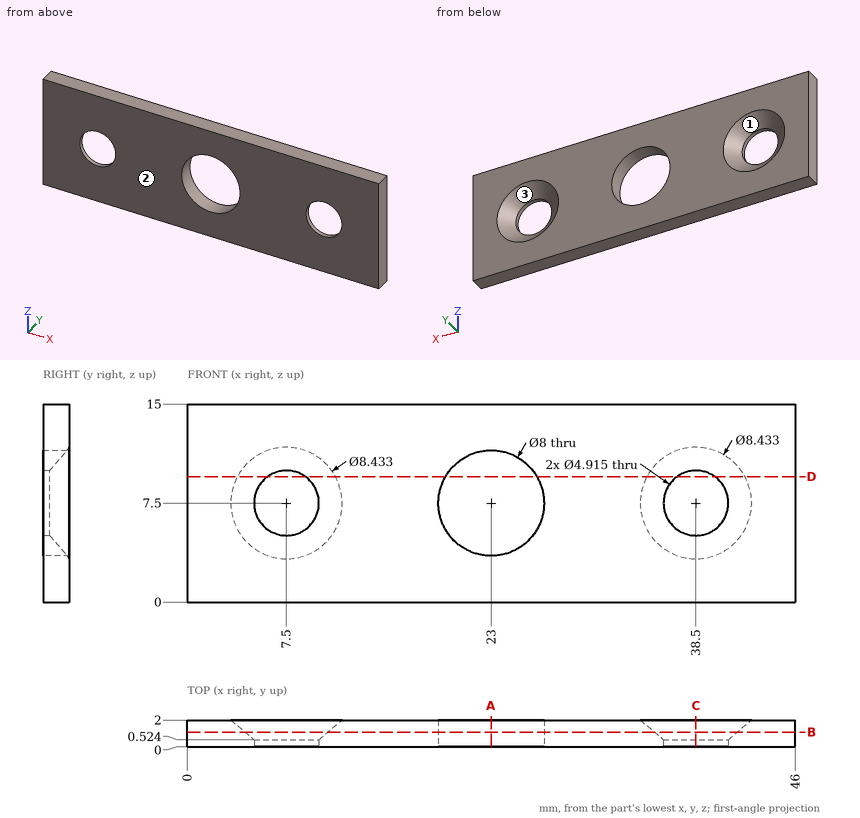
Geometry check sheet. Reference: drawing and pictorial views, mm from the part's lowest x, y, z. Give positions to 0.01 mm unless a question says otherwise; leave off trailing zeros. Loops run counter-clockwise (first coordinate to the right, second up) from the corner with the lowest first, then second, coordinate; pieces in that order, holes last. Notation, with made-up numbers: (69, -30.75) - (90, -30.75) arc R29 ccw to (90, -6.75) - close; hole circle Ø4 at (-2, 88.25). An arc over 180 degrees is marked (long way). One line per question, with ' | ' between items. Start each with the question number.
1. Gauge pin test, flat end, axial feed: pin 1 Ø3 at (x, z) = (7.5, 7.5) entering from +Y. Record the tip position at first contact, or that the pin passes through.
2. Cross-section at C-C, the plane x = 38.5. Enter the section's corners in (y, z), plus the area to 3 significant figures.
3. Cross-section at A-A, the plane x = 23. Enter the section's corners in (y, z).
4. Cross-section at D-D, the plane z = 9.5. Give the number of separate pieces and of enclosed holes in the cut face.
5. Material ranges on line 1 along Z through (x, y) = (7.5, 0.35); line 2 along X through (y, z) = (1.05, 4.25); line 3 along Z through (x, y) = (42, 1.9), recorded low to high. Write a range as [from, to].
6. Draft check along Z on the marked faces 1, 2 and 3. Enter one of: released by +Z, released by -Z, zero draft, split by the parting line, or undercut.
7. Cross-section at B-B, the plane y = 1.1. Enter the section's corners in (x, z).
Check result:
1) pin 1: passes through
2) outline: (0, 0) - (2, 0) - (2, 3.28) - (0.52, 5.04) - (0, 5.04) - close; (0, 9.96) - (0.52, 9.96) - (2, 11.72) - (2, 15) - (0, 15) - close | area: 17.6 mm2
3) outline: (0, 0) - (2, 0) - (2, 3.5) - (0, 3.5) - close; (0, 11.5) - (2, 11.5) - (2, 15) - (0, 15) - close
4) separate pieces: 4 | enclosed holes: 0
5) line 1: z = [0, 5.04], [9.96, 15] | line 2: x = [0, 20.67], [25.33, 46] | line 3: z = [0, 5.37], [9.63, 15]
6) face 1: undercut | face 2: zero draft | face 3: undercut
7) outline: (0, 0) - (46, 0) - (46, 15) - (0, 15) - close; hole circle Ø6.29 at (7.5, 7.5); hole circle Ø8 at (23, 7.5); hole circle Ø6.29 at (38.5, 7.5)
